Part model, mm, in its own coordinate system. A direction names the side the tool comes from. Coordinates: 2 decimals unless noted, no trailing zeros. Loops run counter-clockwise (first coordinate to the right, second up) from the corner with the lowest first, then second, coordinate; pieces in that order, holes last. Notation, with made-up numbers: (4, 82) - (26, 82) arc R10 cw to (26, 98) - close; hole circle Ø9 at (-12.75, -31.5). An arc over 180 degrees is marked (long way). Use a Markdown table: item, result. Add a question column.
1) Band-saw the part on B-B (z = 2.5). Give the cut face in (x, y).
2) Probe probe 1 along Y at (x, z) = (2.7, 2.5); probe 2 along Y at (x, z) = (50, 3.05); probe 3 along X at (y, z) = (3.25, 4.55). List the from-to ranges inside material, lowest first. Write a range as [from, to].
3) Pull direction Y, two halves, no side cores. Call faces 3 (the face through (29, 0, 5)), 4 (the face through (2.465, -1.952, 2.066)), 5 (the face through (25, -8, 2)): +Y half, -Y half, draft (parallel to the pull), parting line (faces both ways), or undercut.
4) Tool access for faces 1 (the face through (5, 0, 2)), 2 (the face through (58, 0, 2)): list every direction of +Z, -Z, +X, -X, +Y, -Y with a clear straight run to the whole face (end or side of a thin tool).
5) Band-saw the part on D-D (y = 2.5). Give the cut face in (x, z).
6) Band-saw the part on C-C (x = 52). Give the cut face in (y, z).
7) Band-saw the part on A-A (y = 0). Give the cut face in (x, z), plus the area to 3 significant figures.
from build123d import *

# Parameters (mm, degrees)
SKETCH1_R           = 4
BOSS_EXTRUDE1_DEPTH = 5
SKETCH2_W           = 5
SKETCH2_H           = 16
CUT_EXTRUDE1_DEPTH  = 59.762232769
SKETCH3_R           = 2
CUT_EXTRUDE3_DEPTH  = 5


with BuildPart() as part:
    # Sketch1 → Boss-Extrude1 (new body)
    with BuildSketch(Plane.XY):
        with BuildLine():
            Line((-50, -8), (50, -8))
            ThreePointArc((50, -8), (58, 0), (50, 8))
            Line((50, 8), (-50, 8))
            ThreePointArc((-50, 8), (-58, 0), (-50, -8))
        make_face()
        with Locations((-50, 0)):
            Circle(SKETCH1_R, mode=Mode.SUBTRACT)
        with Locations((50, 0)):
            Circle(SKETCH1_R, mode=Mode.SUBTRACT)
    extrude(amount=BOSS_EXTRUDE1_DEPTH)

    # Sketch2 → Cut-Extrude1 (cut, through all)
    with BuildSketch(Plane(origin=(0, 0, 0), x_dir=(0, 0, -1), z_dir=(1, 0, 0))):
        with Locations((-2.5, 0)):
            Rectangle(SKETCH2_W, SKETCH2_H)
    extrude(amount=-CUT_EXTRUDE1_DEPTH, mode=Mode.SUBTRACT)

    # Sketch3 → Cut-Extrude3 (cut)
    with BuildSketch(Plane.ZY):
        with Locations((2.5, 0)):
            Circle(SKETCH3_R)
    extrude(amount=-CUT_EXTRUDE3_DEPTH, mode=Mode.SUBTRACT)


solid = part.part
Answer block:
| question | item | result |
|---|---|---|
| 1 | outline | (0, -8) - (50, -8) arc R8 ccw to (50, 8) - (0, 8) - (0, 2) - (5, 2) - (5, -2) - (0, -2) - close; hole circle Ø8 at (50, 0) |
| 2 | probe 1 | [-8, -2], [2, 8] |
| 2 | probe 2 | [-8, -4], [4, 8] |
| 2 | probe 3 | [0, 47.67], [52.33, 57.31] |
| 3 | face 3 | draft |
| 3 | face 4 | undercut |
| 3 | face 5 | -Y half |
| 4 | face 1 | -X |
| 4 | face 2 | +Z, -Z, +X |
| 5 | outline | (0, 0) - (46.88, 0) - (46.88, 5) - (0, 5) - close; (53.12, 0) - (57.6, 0) - (57.6, 5) - (53.12, 5) - close |
| 6 | outline | (-7.75, 0) - (-3.46, 0) - (-3.46, 5) - (-7.75, 5) - close; (3.46, 0) - (7.75, 0) - (7.75, 5) - (3.46, 5) - close |
| 7 | outline | (0, 0) - (46, 0) - (46, 5) - (0, 5) - (0, 4.5) - (5, 4.5) - (5, 0.5) - (0, 0.5) - close; (54, 0) - (58, 0) - (58, 5) - (54, 5) - close |
| 7 | area | 230 mm2 |
